The listing builds one solid part. Answer for the finished solid, in the listing's coordinates (mm). Face numbers are marked on the shaded views. A direction names the side the tool comes from. Round coordinates to 2 decimals unless told otherwise and drop trailing zeros. Loops run counter-clockwise (first coordinate to the right, second up) from the corner with the lowest first, then second, coordinate; pieces in that order, holes last. Notation, with made-up numbers: (6, 1.25) -> (34, 1.25) arc R30 cw to (34, 33.25) -> close; hole circle Ø3 at (67.5, 14.25). An arc over 180 degrees is marked (long way). Use a Markdown table: item, result. Add a question column.
Q1. Given pin 1 Ø1 at (x, y) = (-20.5, 89.5) entering from -Z (3 decimals), flat-ended and moving along its own axis, determine where the tip first touches the part or whether it passes through.
Q2. Section B-B on z = -31 is taken. Give the vertices of the cut face in (x, y) (3 decimals), then the cut area to 3 significant figures.
Q3. Which of the six approach directions +Z, -Z, +X, -X, +Y, -Y give full straight-line access (tool end or side, diameter ignored) to the marked faces 1 and 2?
Q4. Section C-C on y = 33 is taken. Give the vertices of the cut face in (x, z) (3 decimals), then the cut area to 3 significant figures.
Q5. For a pull along Z with two mould halves and no side action, classify the marked faces 3, 4, 5 and 6 as released by +Z, released by -Z, zero draft, split by the parting line, or undercut.
Q6. Consider line 1 (X direction, y = 34, z = -24.5) (3 decimals); line 2 (Z direction, x = -19.5, y = 19) (3 decimals); line 3 (Z direction, x = -20.5, y = 80.5) (3 decimals). Determine where each line is inside the solid, lowest interval first.
Q7. Section A-A on x = -16.5 is taken. Give the vertices of the cut face in (y, z) (3 decimals).
Q8. Section D-D on y = 108 is taken. Give the vertices of the cut face in (x, z) (3 decimals).
Autodesk Inventor part; units mm, degrees
ref_plane "YZ Plane" through (0, 0, 0) normal (1, 0, 0) x (0, 1, 0)
ref_plane "XZ Plane" through (0, 0, 0) normal (0, 1, 0) x (-1, 0, 0)
ref_plane "XY Plane" through (0, 0, 0) normal (0, 0, 1) x (1, 0, 0)
sketch "Sketch1" plane through (0, 0, 0) normal (0, 1, 0) x (-1, 0, 0)
  line L0 (0, 0) -> (25.4, 0)
  line L1 (25.4, 0) -> (25.4, -50.8)
  line L2 (25.4, -50.8) -> (0, -50.8)
  line L3 (0, -50.8) -> (0, 0)
  line L4 (22.225, -47.625) -> (22.225, -3.175)
  line L5 (22.225, -3.175) -> (3.175, -3.175)
  line L6 (3.175, -3.175) -> (3.175, -47.625)
  line L7 (3.175, -47.625) -> (22.225, -47.625)
  dimension "d0" = 25.4
  dimension "d1" = 50.8
  dimension "d2" = 3.175
extrude "Extrusion1" add sketch "Sketch1" along normal blind 75.4888
sketch "Sketch2" plane through (0, 0, 0) normal (1, 0, 0) x (0, 0, -1)
  line L0 (50.8, 0) -> (0, 0)
  line L1 (50.8, 0) -> (50.8, 75.4888)
  line L2 (0, 75.4888) -> (50.8, 75.4888)
  line L3 (0, 0) -> (0, 75.4888)
  line L4 (50.8, 75.4888) -> (0, 131.9079)
  line L5 (0, 131.9079) -> (0, 75.4888)
  dimension "d5" = 48
extrude "Extrusion2" add sketch "Sketch2" against normal blind 25.4 contours L2 L5 L4
sketch "Sketch3" plane through (0, 0, 0) normal (0, -1, 0) x (1, 0, 0)
  line L0 (-22.225, -47.625) -> (-3.175, -47.625)
  line L1 (-3.175, -47.625) -> (-3.175, -3.175)
  line L2 (-3.175, -3.175) -> (-22.225, -3.175)
  line L3 (-22.225, -3.175) -> (-22.225, -47.625)
  point P0 (0, 0)
extrude "Extrusion3" cut sketch "Sketch3" against normal through all
sketch "Sketch4" plane through (0, 0, 0) normal (0, -1, 0) x (1, 0, 0)
  line L0 (-3.175, -47.625) -> (-22.225, -47.625)
  line L1 (-22.225, -47.625) -> (-22.225, -3.175)
  line L2 (-22.225, -3.175) -> (-3.175, -3.175)
  line L3 (-3.175, -3.175) -> (-3.175, -47.625)
  line L4 (0, 0) -> (-25.4, 0)
  line L5 (-25.4, 0) -> (-25.4, -50.8)
  line L6 (-25.4, -50.8) -> (0, -50.8)
  line L7 (0, -50.8) -> (0, 0)
extrude "Extrusion4" add sketch "Sketch4" along normal blind 25.4
properties part number "SmallAnglesSupport.ver1-1111-2020"
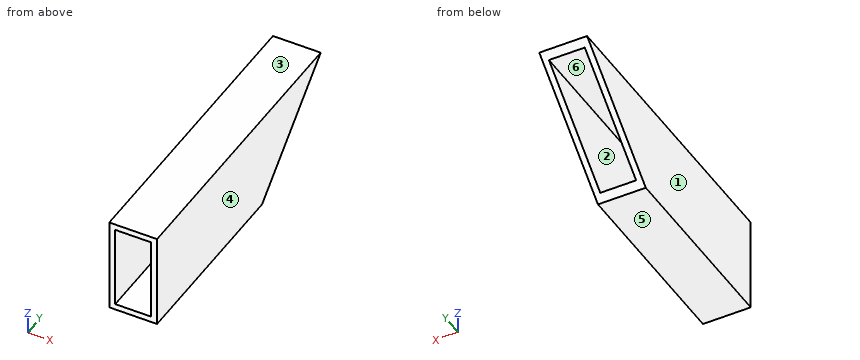
Checked values:
| question | item | result |
|---|---|---|
| 1 | pin 1 | stops at z = -3.175 |
| 2 | outline | (-25.4, -25.4) -> (-22.225, -25.4) -> (-22.225, 97.479) -> (-25.4, 97.479) -> close; (-3.175, -25.4) -> (0, -25.4) -> (0, 97.479) -> (-3.175, 97.479) -> close |
| 2 | area | 780 mm2 |
| 3 | face 1 | +Z, -Z, -X, +Y, -Y |
| 3 | face 2 | +Y, -Y |
| 4 | outline | (-25.4, -50.8) -> (0, -50.8) -> (0, 0) -> (-25.4, 0) -> close; hole (-22.225, -47.625) -> (-3.175, -47.625) -> (-3.175, -3.175) -> (-22.225, -3.175) -> close |
| 4 | area | 444 mm2 |
| 5 | face 3 | released by +Z |
| 5 | face 4 | zero draft |
| 5 | face 5 | released by -Z |
| 5 | face 6 | undercut |
| 6 | line 1 | x = -25.4 to -22.225, -3.175 to 0 |
| 6 | line 2 | z = -50.8 to -47.625, -3.175 to 0 |
| 6 | line 3 | z = -3.175 to 0 |
| 7 | outline | (-25.4, -50.8) -> (75.489, -50.8) -> (79.015, -47.625) -> (-25.4, -47.625) -> close; (-25.4, -3.175) -> (128.382, -3.175) -> (131.908, 0) -> (-25.4, 0) -> close |
| 8 | outline | (-25.4, -21.527) -> (-22.225, -21.527) -> (-22.225, -3.175) -> (-3.175, -3.175) -> (-3.175, -21.527) -> (0, -21.527) -> (0, 0) -> (-25.4, 0) -> close |
